Source: CAD feature listing. Evaluate the final solid. Frame: model axes, mm. A direction names the side the tool comes from. Coordinates: 2 decimals unless noted, no trailing zeros. Loops run counter-clockwise (first coordinate to the right, second up) from the corner with the lowest first, then second, coordinate; pieces in that order, holes last.
Item 1: Pin query (flat end, axial travel): pin 1 Ø12 at (x, z) = (-2, 1) entering from +Y; pin 2 Ø1.5 at (x, z) = (21, 42) entering from +Y; pin 3 Ø6 at (y, z) = (34, -4.5) entering from -X. Return the tip coordinate at first contact, or that it passes through.
Item 2: Section query A-A, the plane y = 16. Return the cut outline in (x, z) (3 decimals), then the cut area to 3 significant figures.
Item 3: Pull-direction query (X, two-part tool) for faces 1 (the flat face through (-42, 38.1, 22)), 2 (the flat face through (42.662, 18.783, -25.093)), 3 (the flat face through (40.192, 25.578, -22.774)); classes: +X half, -X half, draft (parallel to the pull), parting line (faces both ways), or undercut.
Item 4: Section query D-D, the plane z = -28. Return the cut outline in (x, y).
Item 5: Section query B-B, the plane x = -10. Return the cut outline in (y, z), then the cut area to 3 significant figures.
Item 6: Section query C-C, the plane y = 6.5. Return the cut outline in (x, z) (3 decimals), then the cut area to 3 significant figures.
Item 7: Reachability of faces 4 (the flat face through (-43.063, 18.783, -24.4)), 5 (the flat face through (0, 26, -46.194)) from +Z, -Z, +X, -X, +Y, -Y: full face, straight path, thin tool, end or side. Return the list, or none.
Item 8: Line query: probe 1 along Z at (x, y) = (-6, 31); probe 2 along Y at (x, z) = (41, 11); probe 3 along X at (y, z) = (22.5, 28). Output: solid intervals per line, ascending.
Autodesk Inventor part; units mm, degrees
ref_plane "YZ Plane" through (0, 0, 0) normal (1, 0, 0) x (0, 1, 0)
ref_plane "XZ Plane" through (0, 0, 0) normal (0, 1, 0) x (-1, 0, 0)
ref_plane "XY Plane" through (0, 0, 0) normal (0, 0, 1) x (1, 0, 0)
sketch "Sketch1" plane through (0, 0, 0) normal (0, 1, 0) x (-1, 0, 0)
  line L0 (57.15, 0) -> (28.575, 49.4934)
  line L1 (28.575, 49.4934) -> (-28.575, 49.4934)
  line L2 (-28.575, 49.4934) -> (-57.15, 0)
  line L3 (57.15, 0) -> (28.575, -49.4934)
  line L4 (28.575, -49.4934) -> (-28.575, -49.4934)
  line L5 (-28.575, -49.4934) -> (-57.15, 0)
  point P0 (0, 0)
  dimension "d0" = 57.15
  dimension "d1" = 57.15
  dimension "d2" = 57.15
  dimension "d3" = 57.15
extrude "Extrusion1" add sketch "Sketch1" along normal blind 38.1
sketch "Sketch2" plane through (0, 38.1, 0) normal (0, 1, 0) x (1, 0, 0)
  line L0 (0, 0) -> (-53.34, 0)
  line L1 (-53.34, 0) -> (-26.67, -46.1938)
  line L2 (-26.67, -46.1938) -> (26.67, -46.1938)
  line L3 (26.67, -46.1938) -> (53.34, 0)
  line L4 (53.34, 0) -> (26.67, 46.1938)
  line L5 (26.67, 46.1938) -> (-26.67, 46.1938)
  line L6 (-26.67, 46.1938) -> (-53.34, 0)
  dimension "d6" = 53.34
  dimension "d7" = 53.34
  dimension "d8" = 60
  dimension "d9" = 53.34
  dimension "d10" = 53.34
extrude "Extrusion2" cut sketch "Sketch2" against normal blind 31.75
sketch "Sketch3" plane through (0, 6.35, 0) normal (0, 1, 0) x (1, 0, 0)
  line L0 (26.67, -46.1938) -> (-26.67, -46.1938)
  line L1 (-26.67, -46.1938) -> (26.67, -46.1938)
  line L2 (53.34, 0) -> (26.67, -46.1938)
  line L3 (26.67, -46.1938) -> (53.34, 0)
  line L4 (-26.67, 46.1938) -> (26.67, 46.1938)
  line L5 (53.34, 0) -> (26.67, 46.1938)
  line L6 (26.67, 46.1938) -> (-26.67, 46.1938)
  line L7 (-26.67, 46.1938) -> (-53.34, 0)
  line L8 (-26.67, -46.1938) -> (-53.34, 0)
  line L9 (-53.34, 0) -> (-26.67, -46.1938)
  line L10 (-26.67, -46.1938) -> (26.67, -46.1938)
  point P0 (0, 0)
extrude "Extrusion3" add sketch "Sketch3" along normal blind 6.35
sketch "Sketch4" plane through (0, 12.7, 0) normal (0, 1, 0) x (1, 0, 0)
  circle A0 centre (-20.955, -41.7438) radius 1.5
  line L0 (26.67, -46.1938) -> (-26.67, -46.1938)
  circle A1 centre (20.955, -41.7438) radius 1.5
  circle A2 centre (-20.955, 2.7412) radius 1.5
  circle A3 centre (20.955, 2.7412) radius 1.5
  point P0 (0, 0)
  dimension "d15" = 3
  dimension "d16" = 4.45
  dimension "d17" = 3
  dimension "d18" = 41.91
  dimension "d19" = 20.955
  dimension "d20" = 4.45
  dimension "d21" = 3
  dimension "d22" = 44.485
  dimension "d23" = 20.955
  dimension "d24" = 3
  dimension "d25" = 41.91
  dimension "d26" = 44.485
extrude "Extrusion4" cut sketch "Sketch4" against normal blind 8.4667
properties part number "Internal Base"
Verdict:
1. pin 1: stops at y = 12.7
1. pin 2: stops at y = 4.23
1. pin 3: stops at x = -56.28
2. outline: (-57.15, 0) - (-28.575, -49.493) - (28.575, -49.493) - (57.15, 0) - (28.575, 49.493) - (-28.575, 49.493) - close; hole (-53.34, 0) - (-26.67, -46.194) - (26.67, -46.194) - (53.34, 0) - (26.67, 46.194) - (-26.67, 46.194) - close
2. area: 1,090 mm2
3. face 1: draft
3. face 2: +X half
3. face 3: undercut
4. outline: (-40.98, 0) - (40.98, 0) - (40.98, 38.1) - (37.17, 38.1) - (37.17, 12.7) - (-37.17, 12.7) - (-37.17, 38.1) - (-40.98, 38.1) - close
5. outline: (0, -49.49) - (38.1, -49.49) - (38.1, -46.19) - (12.7, -46.19) - (12.7, 46.19) - (38.1, 46.19) - (38.1, 49.49) - (0, 49.49) - close
5. area: 1,420 mm2
6. outline: (-57.15, 0) - (-28.575, -49.493) - (28.575, -49.493) - (57.15, 0) - (28.575, 49.493) - (-28.575, 49.493) - close; hole circle Ø3 at (-20.955, -2.741); hole circle Ø3 at (-20.955, 41.744); hole circle Ø3 at (20.955, -2.741); hole circle Ø3 at (20.955, 41.744)
6. area: 8,460 mm2
7. face 4: -Z, -X, +Y, -Y
7. face 5: +Y
8. probe 1: z = -49.49 to -46.19, 46.19 to 49.49
8. probe 2: y = 0 to 12.7
8. probe 3: x = -40.98 to -37.17, 37.17 to 40.98
